For this review, take the finished solid that the model builds, in its own axes (mm). Coordinates: 2 decimals unless noted, no trailing zeros. Use a Markdown table: item, result.
from build123d import *

# Parameters (mm, degrees)
BOSS_EXTRUDE1_DEPTH    = 300
CUT_EXTRUDE1_OUTLINE_R = 2.5
CUT_EXTRUDE1_DEPTH     = 300


# Read off the part's stored shape, not the designer's step: Cut-Extrude1
with BuildPart() as part:
    # Sketch1 → Boss-Extrude1 (new body)
    with BuildSketch(Plane.XY):
        with BuildLine():
            ThreePointArc((-4.339541497, 3.27832502), (-4.01438237, 2.791689997), (-3.900201668, 2.217664848))
            Line((-3.900201668, 2.217664848), (-3.900201668, -2.220777458))
            ThreePointArc((-3.900201668, -2.220777458), (-4.013982246, -2.793835668), (-4.338062619, -3.279956687))
            ThreePointArc((-4.338062619, -3.279956687), (-4.338801799, -3.280697416), (-4.339541497, -3.28143763))
            Line((-4.339541497, -3.28143763), (-6.559305445, -5.501201578))
            Line((-6.559305445, -5.501201578), (-7.918645273, -5.501201578))
            ThreePointArc((-7.918645273, -5.501201578), (-8.116635172, -5.419191476), (-8.198645273, -5.221201578))
            Line((-8.198645273, -5.221201578), (-8.198645273, -3.381201578))
            ThreePointArc((-8.198645273, -3.381201578), (-8.280655374, -3.183211679), (-8.478645273, -3.101201578))
            Line((-8.478645273, -3.101201578), (-9.418645273, -3.101201578))
            ThreePointArc((-9.418645273, -3.101201578), (-9.616635172, -3.183211679), (-9.698645273, -3.381201578))
            Line((-9.698645273, -3.381201578), (-9.698645273, -3.601201578))
            Line((-9.698645273, -3.601201578), (-9.718645273, -3.601201578))
            ThreePointArc((-9.718645273, -3.601201578), (-9.916635172, -3.683211679), (-9.998645273, -3.881201578))
            Line((-9.998645273, -3.881201578), (-9.998645273, -8.501201578))
            ThreePointArc((-9.998645273, -8.501201578), (-9.559305445, -9.561861749), (-8.498645273, -10.001201578))
            Line((-8.498645273, -10.001201578), (-3.878645273, -10.001201578))
            ThreePointArc((-3.878645273, -10.001201578), (-3.680655374, -9.919191476), (-3.598645273, -9.721201578))
            Line((-3.598645273, -9.721201578), (-3.598645273, -9.701201578))
            Line((-3.598645273, -9.701201578), (-3.378645273, -9.701201578))
            ThreePointArc((-3.378645273, -9.701201578), (-3.180655374, -9.619191476), (-3.098645273, -9.421201578))
            Line((-3.098645273, -9.421201578), (-3.098645273, -8.481201578))
            ThreePointArc((-3.098645273, -8.481201578), (-3.180655374, -8.283211679), (-3.378645273, -8.201201578))
            Line((-3.378645273, -8.201201578), (-5.218645273, -8.201201578))
            ThreePointArc((-5.218645273, -8.201201578), (-5.416635172, -8.119191476), (-5.498645273, -7.921201578))
            Line((-5.498645273, -7.921201578), (-5.498645273, -6.561861749))
            Line((-5.498645273, -6.561861749), (-3.277324929, -4.340541406))
            ThreePointArc((-3.277324929, -4.340541406), (-2.790689906, -4.015382279), (-2.216664757, -3.901201578))
            Line((-2.216664757, -3.901201578), (2.234977304, -3.899793498))
            ThreePointArc((2.234977304, -3.899793498), (2.801097117, -4.016727825), (3.280957809, -4.339061494))
            Line((3.280957809, -4.339061494), (5.502201668, -6.560305354))
            Line((5.502201668, -6.560305354), (5.502201668, -7.919645182))
            ThreePointArc((5.502201668, -7.919645182), (5.420191567, -8.117635081), (5.222201668, -8.199645182))
            Line((5.222201668, -8.199645182), (3.382201668, -8.199645182))
            ThreePointArc((3.382201668, -8.199645182), (3.18421177, -8.281655283), (3.102201668, -8.479645182))
            Line((3.102201668, -8.479645182), (3.102201668, -9.419645182))
            ThreePointArc((3.102201668, -9.419645182), (3.18421177, -9.617635081), (3.382201668, -9.699645182))
            Line((3.382201668, -9.699645182), (3.602201668, -9.699645182))
            Line((3.602201668, -9.699645182), (3.602201668, -9.719645182))
            ThreePointArc((3.602201668, -9.719645182), (3.68421177, -9.917635081), (3.882201668, -9.999645182))
            Line((3.882201668, -9.999645182), (8.502201668, -9.999645182))
            ThreePointArc((8.502201668, -9.999645182), (9.56286184, -9.560305354), (10.002201668, -8.499645182))
            Line((10.002201668, -8.499645182), (10.002201668, -3.879645182))
            ThreePointArc((10.002201668, -3.879645182), (9.920191567, -3.681655283), (9.722201668, -3.599645182))
            Line((9.722201668, -3.599645182), (9.702201668, -3.599645182))
            Line((9.702201668, -3.599645182), (9.702201668, -3.379645182))
            ThreePointArc((9.702201668, -3.379645182), (9.620191567, -3.181655283), (9.422201668, -3.099645182))
            Line((9.422201668, -3.099645182), (8.482201668, -3.099645182))
            ThreePointArc((8.482201668, -3.099645182), (8.28421177, -3.181655283), (8.202201668, -3.379645182))
            Line((8.202201668, -3.379645182), (8.202201668, -5.219645182))
            ThreePointArc((8.202201668, -5.219645182), (8.120191567, -5.417635081), (7.922201668, -5.499645182))
            Line((7.922201668, -5.499645182), (6.56286184, -5.499645182))
            Line((6.56286184, -5.499645182), (4.341541497, -3.278324838))
            ThreePointArc((4.341541497, -3.278324838), (4.01638237, -2.791689815), (3.902201668, -2.217664667))
            Line((3.902201668, -2.217664667), (3.900793589, 2.233977395))
            ThreePointArc((3.900793589, 2.233977395), (4.017727916, 2.800097207), (4.340061585, 3.2799579))
            Line((4.340061585, 3.2799579), (6.561305445, 5.501201759))
            Line((6.561305445, 5.501201759), (7.920645273, 5.501201759))
            ThreePointArc((7.920645273, 5.501201759), (8.118635172, 5.419191658), (8.200645273, 5.221201759))
            Line((8.200645273, 5.221201759), (8.200645273, 3.381201759))
            ThreePointArc((8.200645273, 3.381201759), (8.282655374, 3.183211861), (8.480645273, 3.101201759))
            Line((8.480645273, 3.101201759), (9.420645273, 3.101201759))
            ThreePointArc((9.420645273, 3.101201759), (9.618635172, 3.183211861), (9.700645273, 3.381201759))
            Line((9.700645273, 3.381201759), (9.700645273, 3.601201759))
            Line((9.700645273, 3.601201759), (9.720645273, 3.601201759))
            ThreePointArc((9.720645273, 3.601201759), (9.918635172, 3.683211861), (10.000645273, 3.881201759))
            Line((10.000645273, 3.881201759), (10.000645273, 8.501201759))
            ThreePointArc((10.000645273, 8.501201759), (9.561305445, 9.561861931), (8.500645273, 10.001201759))
            Line((8.500645273, 10.001201759), (3.880645273, 10.001201759))
            ThreePointArc((3.880645273, 10.001201759), (3.682655374, 9.919191658), (3.600645273, 9.721201759))
            Line((3.600645273, 9.721201759), (3.600645273, 9.701201759))
            Line((3.600645273, 9.701201759), (3.380645273, 9.701201759))
            ThreePointArc((3.380645273, 9.701201759), (3.182655374, 9.619191658), (3.100645273, 9.421201759))
            Line((3.100645273, 9.421201759), (3.100645273, 8.481201759))
            ThreePointArc((3.100645273, 8.481201759), (3.182655374, 8.283211861), (3.380645273, 8.201201759))
            Line((3.380645273, 8.201201759), (5.220645273, 8.201201759))
            ThreePointArc((5.220645273, 8.201201759), (5.418635172, 8.119191658), (5.500645273, 7.921201759))
            Line((5.500645273, 7.921201759), (5.500645273, 6.561861931))
            Line((5.500645273, 6.561861931), (3.279324929, 4.340541588))
            ThreePointArc((3.279324929, 4.340541588), (2.792689906, 4.015382461), (2.218664757, 3.901201759))
            Line((2.218664757, 3.901201759), (-2.232977304, 3.89979368))
            ThreePointArc((-2.232977304, 3.89979368), (-2.799097117, 4.016728006), (-3.278957809, 4.339061676))
            Line((-3.278957809, 4.339061676), (-5.500201668, 6.560305535))
            Line((-5.500201668, 6.560305535), (-5.500201668, 7.919645364))
            ThreePointArc((-5.500201668, 7.919645364), (-5.418191567, 8.117635262), (-5.220201668, 8.199645364))
            Line((-5.220201668, 8.199645364), (-3.380201668, 8.199645364))
            ThreePointArc((-3.380201668, 8.199645364), (-3.18221177, 8.281655465), (-3.100201668, 8.479645364))
            Line((-3.100201668, 8.479645364), (-3.100201668, 9.419645364))
            ThreePointArc((-3.100201668, 9.419645364), (-3.18221177, 9.617635262), (-3.380201668, 9.699645364))
            Line((-3.380201668, 9.699645364), (-3.600201668, 9.699645364))
            Line((-3.600201668, 9.699645364), (-3.600201668, 9.719645364))
            ThreePointArc((-3.600201668, 9.719645364), (-3.68221177, 9.917635262), (-3.880201668, 9.999645364))
            Line((-3.880201668, 9.999645364), (-8.500201668, 9.999645364))
            ThreePointArc((-8.500201668, 9.999645364), (-9.56086184, 9.560305535), (-10.000201668, 8.499645364))
            Line((-10.000201668, 8.499645364), (-10.000201668, 3.879645364))
            ThreePointArc((-10.000201668, 3.879645364), (-9.918191567, 3.681655465), (-9.720201668, 3.599645364))
            Line((-9.720201668, 3.599645364), (-9.700201668, 3.599645364))
            Line((-9.700201668, 3.599645364), (-9.700201668, 3.379645364))
            ThreePointArc((-9.700201668, 3.379645364), (-9.618191567, 3.181655465), (-9.420201668, 3.099645364))
            Line((-9.420201668, 3.099645364), (-8.480201668, 3.099645364))
            ThreePointArc((-8.480201668, 3.099645364), (-8.28221177, 3.181655465), (-8.200201668, 3.379645364))
            Line((-8.200201668, 3.379645364), (-8.200201668, 5.219645364))
            ThreePointArc((-8.200201668, 5.219645364), (-8.118191567, 5.417635262), (-7.920201668, 5.499645364))
            Line((-7.920201668, 5.499645364), (-6.56086184, 5.499645364))
            Line((-6.56086184, 5.499645364), (-4.339541497, 3.27832502))
        make_face()
    extrude(amount=BOSS_EXTRUDE1_DEPTH)

    # Cut-Extrude1 outline → Cut-Extrude1 (cut)
    with BuildSketch(Plane.XY):
        Circle(CUT_EXTRUDE1_OUTLINE_R)
    extrude(amount=CUT_EXTRUDE1_DEPTH, mode=Mode.SUBTRACT)


solid = part.part
(1) For pin 1 Ø0.5 at (x, z) = (9, 116) entering from +Y; pin 2 Ø2 at (x, y) = (2, -1.5) entering from -Z; pin 3 Ø0.8 at (y, z) = (-9, 167) entering from +X, all flat-tipped, find the tip position at first contact; note any pin that passes through.
Found:
| item | result |
|---|---|
| pin 1 | stops at y = 9.98 |
| pin 2 | stops at z = 0 |
| pin 3 | stops at x = 10 |
(2) Mouldability with a two-part tool opening along X and no side actions: class faces 1 (the face through (-0.54, -2.44, 147.9)), 2 (the face through (-6, 10, 148)), 3 (the face through (10.001, 6, 148)) as pulls with the +X half, pulls with the -X half, needs draft (parallel to the pull), parting line crosses it, or undercut.
Found:
| item | result |
|---|---|
| face 1 | undercut |
| face 2 | needs draft |
| face 3 | pulls with the +X half |
(3) For line 1 along X through (y, z) = (-4.5, 228); line 2 along X through (y, z) = (-1.25, 264.5); line 3 along Y through (x, z) = (0, 128.5), list the stretches that pass through material, from the lowest coordinate up.
Found:
| item | result |
|---|---|
| line 1 | x = -10 to -8.2, -5.56 to -3.44, 3.44 to 5.56, 8.2 to 10 |
| line 2 | x = -3.9 to -2.17, 2.17 to 3.9 |
| line 3 | y = -3.9 to -2.5, 2.5 to 3.9 |
